Design review of the part built by this model. Coordinates are the model's own, in mm. Give positions to 0.01 mm unless a question says otherwise; leave off trailing zeros. Write each loop counter-clockwise with the first axis right and the second up, starting at its lowest first coordinate (ties: lowest second). Pieces come first, ordered by that corner, then holes. Notation, with made-up numbers: (77, 64.25) -> (98, 64.25) arc R14 cw to (98, 79.25) -> close; hole circle Ø7 at (10.5, -21). An arc over 180 degrees is marked (long way). Answer as a JSON object with one key per item and string values.
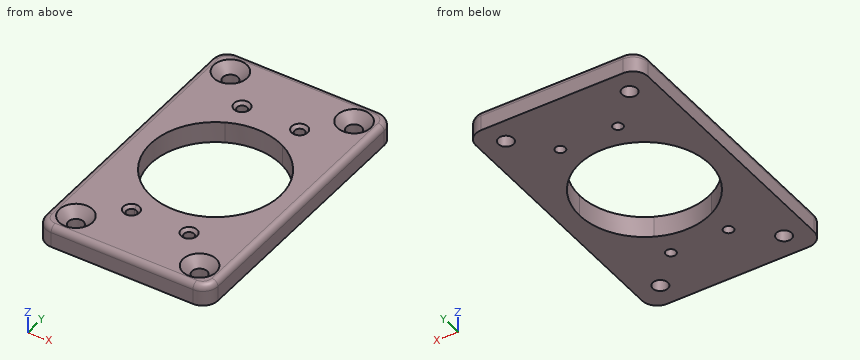
```python
from build123d import *

# Parameters (mm, degrees)
SKETCH1_W           = 57
SKETCH1_H           = 94
SKETCH1_R           = 2.5
SKETCH1_R_2         = 1.65
BOSS_EXTRUDE1_DEPTH = 7
CHAMFER1_SIZE       = 3
FILLET1_R           = 5
FILLET2_R           = 2
CHAMFER2_SIZE       = 1
CUT_EXTRUDE1_DEPTH  = 10


with BuildPart() as part:
    # Sketch1 → Boss-Extrude1 (new body)
    with BuildSketch(Plane.XY):
        with Locations((-18.5, -37)):
            Rectangle(SKETCH1_W, SKETCH1_H)
        with Locations((-39, -76.0375)):
            Circle(SKETCH1_R, mode=Mode.SUBTRACT)
        with BuildLine():
            ThreePointArc((-26.025, -65.25), (-28.841726189, -66.416726189), (-27.675, -63.6))
            ThreePointArc((-27.675, -63.6), (-26.508273811, -64.083273811), (-26.025, -65.25))
        make_face(mode=Mode.SUBTRACT)
        with Locations((-8.575, -65.25)):
            Circle(SKETCH1_R_2, mode=Mode.SUBTRACT)
        with Locations((2, -76.0375)):
            Circle(SKETCH1_R, mode=Mode.SUBTRACT)
        with BuildLine():
            ThreePointArc((-26.025, -9.35), (-26.508273811, -10.516726189), (-27.675, -11))
            ThreePointArc((-27.675, -11), (-28.841726189, -8.183273811), (-26.025, -9.35))
        make_face(mode=Mode.SUBTRACT)
        with Locations((-8.575, -9.35)):
            Circle(SKETCH1_R_2, mode=Mode.SUBTRACT)
        with Locations((2, 2.0375)):
            Circle(SKETCH1_R, mode=Mode.SUBTRACT)
        with Locations((-39, 2.0375)):
            Circle(SKETCH1_R, mode=Mode.SUBTRACT)
    extrude(amount=BOSS_EXTRUDE1_DEPTH)

    # Chamfer1
    chamfer1_edges = [part.edges().sort_by_distance(p)[0] for p in [
        (-0.5, -76.0375, 7),
        (-41.5, -76.0375, 7),
        (-0.5, 2.0375, 7),
        (-41.5, 2.0375, 7),
    ]]
    chamfer(chamfer1_edges, length=CHAMFER1_SIZE)

    # Fillet1
    fillet1_edges = [part.edges().sort_by_distance(p)[0] for p in [
        (10, 10, 3.5),
        (10, -84, 3.5),
        (-47, -84, 3.5),
        (-47, 10, 3.5),
    ]]
    fillet(fillet1_edges, radius=FILLET1_R)

    # Fillet2
    fillet2_edges = [part.edges().sort_by_distance(p)[0] for p in [
        (-18.5, 10, 7),
        (10, -37, 7),
        (-47, -37, 7),
        (-18.5, -84, 7),
        (8.535533906, -82.535533906, 7),
        (-45.535533906, -82.535533906, 7),
        (-45.535533906, 8.535533906, 7),
        (8.535533906, 8.535533906, 7),
    ]]
    fillet(fillet2_edges, radius=FILLET2_R)

    # Chamfer2
    chamfer2_edges = [part.edges().sort_by_distance(p)[0] for p in [
        (-29.325, -9.35, 7),
        (-10.225, -65.25, 7),
        (-27.675, -66.9, 7),
        (-10.225, -9.35, 7),
    ]]
    chamfer(chamfer2_edges, length=CHAMFER2_SIZE)

    # Sketch3 → Cut-Extrude1 (cut)
    with BuildSketch(Plane.XY.offset(7)):
        with BuildLine():
            Line((-27.675, -56.562593283), (-27.675, -18.037406717))
            ThreePointArc((-27.675, -18.037406717), (-39.625, -37.3), (-27.675, -56.562593283))
        make_face()
        with BuildLine():
            ThreePointArc((-8.575, -18.037406717), (-18.125, -15.8), (-27.675, -18.037406717))
            Line((-27.675, -18.037406717), (-27.675, -56.562593283))
            ThreePointArc((-27.675, -56.562593283), (-18.125, -58.8), (-8.575, -56.562593283))
            Line((-8.575, -56.562593283), (-8.575, -18.037406717))
        make_face()
        with BuildLine():
            ThreePointArc((3.375, -37.3), (0.144852216, -25.965870126), (-8.575, -18.037406717))
            Line((-8.575, -18.037406717), (-8.575, -56.562593283))
            ThreePointArc((-8.575, -56.562593283), (0.144852216, -48.634129874), (3.375, -37.3))
        make_face()
    extrude(amount=-CUT_EXTRUDE1_DEPTH, mode=Mode.SUBTRACT)


solid = part.part
```
(1) We need section D-D, the plane z = 1. Give the number of separate pieces and of enclosed holes in the cut face, then the cut area to 3 significant figures.
Here are the results:
{"separate pieces": "1", "enclosed holes": "9", "area": "3,770 mm²"}
(2) Clearance check with flat-ended pins moving along their axes: pin 1 (4 mm diameter, centred on x = -39, y = 2.04, fed in from +Z); pin 2 (4.5 mm diameter, centred on x = -27.675, y = -65.25, fed in from +Z); pin 3 (6.5 mm diameter, centred on x = 2, y = 2.04, fed in from +Z). State where each tip first meets the part, or that it passes through.
Here are the results:
{"pin 1": "passes through", "pin 2": "stops at z = 6.6", "pin 3": "stops at z = 4.75"}
(3) We need section C-C, the plane x = 2. State the section outline as (y, z) points.
Here are the results:
{"outline": "(-84, 0) -> (-78.54, 0) -> (-78.54, 4) -> (-81.54, 7) -> (-82, 7) arc R2 ccw to (-84, 5) -> close; (-73.54, 0) -> (-44.87, 0) -> (-44.87, 7) -> (-70.54, 7) -> (-73.54, 4) -> close; (-29.73, 0) -> (-0.46, 0) -> (-0.46, 4) -> (-3.46, 7) -> (-29.73, 7) -> close; (4.54, 0) -> (10, 0) -> (10, 5) arc R2 ccw to (8, 7) -> (7.54, 7) -> (4.54, 4) -> close"}
(4) We need section A-A, the plane x = -21.5. State the section outline as (y, z) points.
Here are the results:
{"outline": "(-84, 0) -> (-58.53, 0) -> (-58.53, 7) -> (-82, 7) arc R2 ccw to (-84, 5) -> close; (-16.07, 0) -> (10, 0) -> (10, 5) arc R2 ccw to (8, 7) -> (-16.07, 7) -> close"}
(5) We need section B-B, the plane y = -54.5. State the section outline as (x, z) points (3 decimals), then the cut area to 3 significant figures.
Here are the results:
{"outline": "(-47, 0) -> (-31.025, 0) -> (-31.025, 7) -> (-45, 7) arc R2 ccw to (-47, 5) -> close; (-5.225, 0) -> (10, 0) -> (10, 5) arc R2 ccw to (8, 7) -> (-5.225, 7) -> close", "area": "217 mm²"}
(6) For line 1 along X through (y, z) = (-65.25, 3.25) (3 decimals); line 2 along X through (y, z) = (-77, 2.75); line 3 along Y through (x, z) = (-8, 2.5), list the stretches that pass through material, from the lowest coordinate up.
Here are the results:
{"line 1": "x = -47 to -29.325, -26.025 to -10.225, -6.925 to 10", "line 2": "x = -47 to -41.31, -36.69 to -0.31, 4.31 to 10", "line 3": "y = -84 to -66.8, -63.7 to -56.27, -18.33 to -10.9, -7.8 to 10"}
